```python
from build123d import *

# Parameters (mm, degrees)
F1_DEPTH = 63.5
F0_W     = 24.7683575517
F0_H     = 19.05
F0_H_2   = 4.7498
F0_H_3   = 4.7752
F2_DEPTH = 25.4
F3_DEPTH = 7.9375
F5_R     = 5.08


with BuildPart() as f1:
    # F0 (on Front) → F1 (new body, symmetric)
    with BuildSketch(Plane.XZ):
        Polygon((22.225, 9.525), (-41.275, 9.525), (-41.275, -9.525), (41.275, -9.525), (41.275, 9.525), align=None)
    extrude(amount=F1_DEPTH, both=True)

    # F0 (on Front) → F2 (join, symmetric)
    with BuildSketch(Plane.XZ):
        with BuildLine():
            Line((22.225, 27.0002), (22.225, 9.525))
            Line((22.225, 9.525), (41.275, 9.525))
            Line((41.275, 9.525), (41.275, 27.0002))
            ThreePointArc((41.275, 27.0002), (45.9246798487, 38.2255201513), (57.15, 42.8752))
            Line((57.15, 42.8752), (60.9566424483, 42.8752))
            Line((60.9566424483, 42.8752), (60.9566424483, 61.9252))
            Line((60.9566424483, 61.9252), (57.15, 61.9252))
            ThreePointArc((57.15, 61.9252), (32.4542956671, 51.6959043329), (22.225, 27.0002))
        make_face()
        with Locations((73.3408212242, 52.4002)):
            Rectangle(F0_W, F0_H)
        with Locations((73.3408212242, 64.3001)):
            Rectangle(F0_W, F0_H_2)
        with Locations((73.3408212242, 40.4876)):
            Rectangle(F0_W, F0_H_3)
        Polygon((85.725, 66.675), (85.725, 61.9252), (85.725, 42.8752), (85.725, 38.1), (111.7566424483, 38.1), (111.7566424483, 66.675), align=None)
    extrude(amount=F2_DEPTH, both=True)

    # F0 (on Front) → F3 (join, symmetric)
    with BuildSketch(Plane.XZ):
        with BuildLine():
            add(Edge.make_bspline(
                [(-41.275, 9.525), (-16.9699750841, 40.0587767363), (10.705399327, 62.3685158789), (57.15, 61.9252)],
                knots=[0, 0, 0, 0, 111.5045361635, 111.5045361635, 111.5045361635, 111.5045361635], degree=3))
            Line((-41.275, 9.525), (22.225, 9.525))
            Line((22.225, 9.525), (22.225, 27.0002))
            ThreePointArc((22.225, 27.0002), (32.4542956671, 51.6959043329), (57.15, 61.9252))
        make_face()
    extrude(amount=F3_DEPTH, both=True)

    # F0 (on Front) → F4 (revolve)
    with BuildSketch(Plane.XZ):
        with Locations((73.3408212242, 64.3001)):
            Rectangle(F0_W, F0_H_2)
        Polygon((85.725, 66.675), (85.725, 61.9252), (85.725, 42.8752), (85.725, 38.1), (111.7566424483, 38.1), (111.7566424483, 66.675), align=None)
        with Locations((73.3408212242, 40.4876)):
            Rectangle(F0_W, F0_H_3)
    revolve(axis=Axis((111.7566424483, 0, 52.3875), (0, 0, 1)))

    # F5
    f5_edges = [f1.edges().sort_by_distance(p)[0] for p in [
        (41.275, -63.5, 0),
        (-41.275, -63.5, 0),
        (-41.275, 63.5, 0),
        (41.275, 63.5, 0),
    ]]
    fillet(f5_edges, radius=F5_R)


solid = f1.part
```
Geometry check sheet. Reference: the model listing, model coordinates, mm. A direction names the side the tool comes from. Round coordinates to 2 decimals unless told otherwise and drop trailing zeros. Loops run counter-clockwise (first coordinate to the right, second up) from the corner with the lowest first, then second, coordinate; pieces in that order, holes last. Notation, with made-up numbers: (37.5, 57.25) - (80.5, 57.25) arc R14 ccw to (80.5, 70.25) - close; hole circle Ø2 at (67, 67). An arc over 180 degrees is marked (long way). Write each question's results on one line, items separated by ' | '. Start each with the question number.
Q1. Cross-section at B-B on z = -1.5. Enter the section's corners in (x, y) (3 decimals), and give its area (3 significant figures).
Q2. Access from +Z, -Z, +X, -X, +Y, -Y to the whole of each face (thin tool, end or side, straight path). Record for faces 1 (the flat face through (9, 7.938, 30)), 2 (the flat face through (59, 0, 61.925)), 3 (the flat face through (59, 0, 42.875)), 4 (the cylindrical face through (32.73, -16.79, 51.97)).
Q3. Cross-section at A-A on y = -35. Enter the section's corners in (x, z) (3 decimals), and give its area (3 significant figures).
Q4. Thickness scan on line 1 (Z direction, x = 86.5, y = 29) (3 decimals); line 2 (Z direction, x = 39, y = 52) (3 decimals); line 3 (Y direction, x = 29.5, z = 38.5). Record the ranges inside material, lowest first. Write a range as [from, to].
Q5. Cross-section at D-D on y = -53. Enter the section's corners in (x, z) (3 decimals), and give its area (3 significant figures).
Q6. Gauge pin test, flat ends, axial feed: P1, Ø1.1, axis at x = 59, y = 3, coming from the -Z side; P2, Ø1.9, axis at x = 58.5, y = 8, coming from the +Z side; P3, Ø4, axis at y = 9.5, z = 64.5, coming from the -X side; P4, Ø19, axis at y = 16.5, z = 14.5, coming from the -X side (3 decimals). Record the tip position at first contact, or that the pin passes through.
Q7. Release check for a two-part mould opening along X. For faces 5 (the flat face through (111, -1, 38.1)), 6 (the cylindrical face through (162.523, -1.862, 64.333)), 7 (the cylindrical face through (45.8, -0.4, 38.1)), 8 (the flat face through (60.957, 0, 40)) record: +X half, -X half, draft (parallel to the pull), parting line (faces both ways), or undercut.
Q8. Cross-section at C-C on y = 19. Enter the section's corners in (x, z) (3 decimals).
Answers below:
1) outline: (-41.275, -58.42) arc R5.08 ccw to (-36.195, -63.5) - (36.195, -63.5) arc R5.08 ccw to (41.275, -58.42) - (41.275, 58.42) arc R5.08 ccw to (36.195, 63.5) - (-36.195, 63.5) arc R5.08 ccw to (-41.275, 58.42) - close | area: 10,500 mm²
2) face 1: +Z, -X, +Y | face 2: +Z, -X, +Y, -Y | face 3: -Z, +Y, -Y | face 4: +Z, -X, -Y
3) outline: (-41.275, -9.525) - (41.275, -9.525) - (41.275, 9.525) - (-41.275, 9.525) - close; (74.938, 38.1) - (148.576, 38.1) - (148.576, 42.875) - (74.938, 42.875) - close; (74.938, 61.925) - (148.576, 61.925) - (148.576, 66.675) - (74.938, 66.675) - close | area: 2,270 mm²
4) line 1: z = [38.1, 42.875], [61.925, 66.675] | line 2: z = [-9.525, 9.525] | line 3: y = [-25.4, 25.4]
5) outline: (-41.275, -9.525) - (41.275, -9.525) - (41.275, 9.525) - (-41.275, 9.525) - close | area: 1,570 mm²
6) P1: stops at z = 42.88 | P2: stops at z = 61.93 | P3: stops at x = 60.96 | P4: stops at x = -41.275
7) face 5: draft | face 6: parting line | face 7: undercut | face 8: undercut
8) outline: (-41.275, -9.525) - (41.275, -9.525) - (41.275, 27) arc R15.875 cw to (57.15, 42.875) - (60.957, 42.875) - (60.957, 38.1) - (158.87, 38.1) - (158.87, 42.875) - (129.551, 42.875) - (129.551, 61.925) - (158.87, 61.925) - (158.87, 66.675) - (60.957, 66.675) - (60.957, 61.925) - (57.15, 61.925) arc R34.925 ccw to (22.225, 27) - (22.225, 9.525) - (-41.275, 9.525) - close
